Design review of the part built by this model. Coordinates are the model's own, in mm. A direction names the side the tool comes from. Coordinates: 2 decimals unless noted, no trailing zeros. Write each loop counter-clockwise with the first axis right and the second up, starting at its lowest first coordinate (ties: lowest second). Pieces come first, ordered by that corner, then holes. Notation, with made-up numbers: M 0.25,42.5 L 33.25,42.5 A35 cw 33.25,80.5 Z; hole C 39,61 d5. An arc over 180 degrees is marked long. Write item = value, one per line.
```python
from build123d import *

# Parameters (mm, degrees)
ESQUISSE1_W        = 5
ESQUISSE1_H        = 3
BOSS_EXTRU_1_DEPTH = 3


with BuildPart() as part:
    # Esquisse1 → Boss.-Extru.1 (new body)
    with BuildSketch(Plane.XY):
        with Locations((6.490106642, -1.399569673)):
            Rectangle(ESQUISSE1_W, ESQUISSE1_H)
        with Locations((16.490106642, -1.399569673)):
            Rectangle(ESQUISSE1_W, ESQUISSE1_H)
        Polygon((-1.009893358, 0.100430327), (3.990106642, 0.100430327), (8.990106642, 0.100430327), (13.990106642, 0.100430327), (18.990106642, 0.100430327), (24.990106642, 0.100430327), (24.990106642, 3.100430327), (-1.009893358, 3.100430327), align=None)
    extrude(amount=BOSS_EXTRU_1_DEPTH)


solid = part.part
```
Q1. Consider section B-B, the plane z = 0.65. State the section outline as (x, y) points.
Check result:
outline = M -1.01,0.1 L 3.99,0.1 L 3.99,-2.9 L 8.99,-2.9 L 8.99,0.1 L 13.99,0.1 L 13.99,-2.9 L 18.99,-2.9 L 18.99,0.1 L 24.99,0.1 L 24.99,3.1 L -1.01,3.1 Z
Q2. Consider section A-A, the plane y = -1.9. State the section outline as (x, z) points.
Check result:
outline = M 3.99,0 L 8.99,0 L 8.99,3 L 3.99,3 Z; M 13.99,0 L 18.99,0 L 18.99,3 L 13.99,3 Z
Q3. Machinability: for faces 5 (the flat face through (3.99, -1, 1)), 6 (the flat face through (12, 3.1, 1)), 7 (the flat face through (8.99, -1, 1)), which of the approach directions +Z, -Z, +X, -X, +Y, -Y give a long, thin tool a straight path to every point of the face, cutting with its end or side? Answer none if there is none.
Check result:
face_5 = +Z, -Z, -X, -Y
face_6 = +Z, -Z, +X, -X, +Y
face_7 = +Z, -Z, -Y
Q4. Wall thickness on line 1 (X direction, y = -1.2, z = 0.2); line 2 (Y direction, x = 11.5, z = 2.5): over which ranges is each line inside the solid? List them lowest first.
Check result:
line_1 = 3.99 to 8.99, 13.99 to 18.99
line_2 = 0.1 to 3.1
Q5. For P1, Ø1.5, axis at y = -1, z = 1.5, coming from the -X side; P2, Ø1.5, axis at x = 21.5, z = 2, coming from the -Y side; P3, Ø1.5, axis at x = 13.5, y = 2, coming from the -Z side; P4, Ø1.5, axis at y = -1.5, z = 1.5, coming from the +X side, all flat-tipped, find the tip position at first contact; note any pin that passes through.
Check result:
P1 = 3.99
P2 = 0.1
P3 = 0
P4 = 18.99
Q6. Consider section C-C, the plane x = 22. State the section outline as (y, z) points, and give its area (3 significant figures).
Check result:
outline = M 0.1,0 L 3.1,0 L 3.1,3 L 0.1,3 Z
area = 9.00 mm²
Q7. The part is to be moulded in two halves that separate along X. For faces 1 (the flat face through (-1.01, 2, 1)), 2 (the flat face through (22, 0.1, 1)), 3 (the flat face through (18.99, -1, 1)), 4 (the flat face through (13.99, -1, 1)), say which applies: +X half, -X half, draft (parallel to the pull), parting line (faces both ways), or undercut.
Check result:
face_1 = -X half
face_2 = draft
face_3 = +X half
face_4 = undercut
